Source: CAD feature listing. Evaluate the final solid. Frame: model axes, mm. Face numbers are marked on the shaded views. A direction names the side the tool comes from. Give positions to 0.01 mm unless a question says otherwise; leave off trailing zeros. Loops run counter-clockwise (first coordinate to the right, second up) from the corner with the lowest first, then second, coordinate; pieces in that order, holes last. Notation, with made-up numbers: M 22.25,66 L 46.25,66 A21 ccw 46.25,94 Z; hole C 89,88.25 d1. An arc over 180 degrees is marked long. Answer in a Markdown table with one row per item.
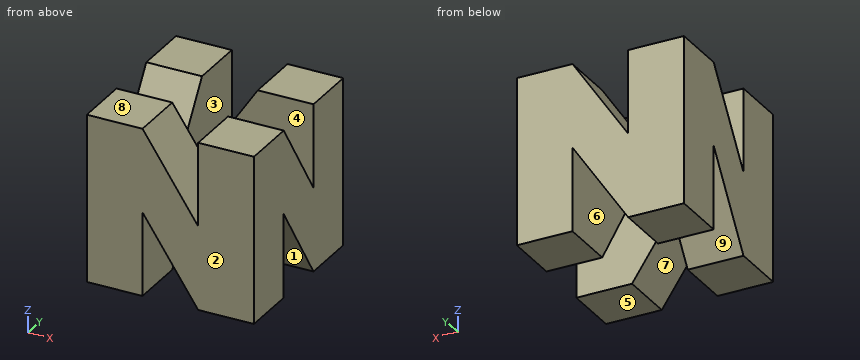
```python
from build123d import *

# Parameters (mm, degrees)
F0_W      = 152.4
F0_H      = 152.4
F1_DEPTH  = 76.2
F2_W      = 25.4
F2_H      = 25.4
F3_DEPTH  = 152.401
F5_DEPTH  = 50.8
F7_DEPTH  = 50.8
F9_DEPTH  = 50.8
F11_DEPTH = 50.8


with BuildPart() as f1:
    # F0 (on Top) → F1 (new body, symmetric)
    with BuildSketch(Plane.XY):
        with Locations((0, 4.4160668929)):
            Rectangle(F0_W, F0_H)
    extrude(amount=F1_DEPTH, both=True)

    # F2 (on face) → F3 (cut, through all)
    with BuildSketch(Plane.XY.offset(76.2)):
        Polygon((0, 29.8160668929), (-25.4, 29.8160668929), (0, 4.4160668929), align=None)
        with Locations((12.7, 17.1160668929)):
            Rectangle(F2_W, F2_H)
        Polygon((25.4, 4.4160668929), (0, 4.4160668929), (25.4, -20.9839331071), align=None)
        Polygon((25.4, -20.9839331071), (0, 4.4160668929), (0, -20.9839331071), align=None)
        with Locations((-12.7, -8.2839331071)):
            Rectangle(F2_W, F2_H)
        Polygon((0, 4.4160668929), (-25.4, 29.8160668929), (-25.4, 4.4160668929), align=None)
    extrude(amount=-F3_DEPTH, mode=Mode.SUBTRACT)

    # F4 (on face) → F5 (cut)
    with BuildSketch(Plane(origin=(0, 80.6160668929, 0), x_dir=(-1, 0, 0), z_dir=(0, 1, 0))):
        Polygon((25.4, -76.2), (-25.4, 0), (-25.4, -76.2), align=None)
        Polygon((25.4, 76.2), (-25.4, 76.2), (25.4, 0), align=None)
    extrude(amount=-F5_DEPTH, mode=Mode.SUBTRACT)

    # F6 (on face) → F7 (cut)
    with BuildSketch(Plane(origin=(-76.2, 0, 0), x_dir=(0, -1, 0), z_dir=(-1, 0, 0))):
        Polygon((20.9839331071, -76.2), (-29.8160668929, 0), (-29.8160668929, -76.2), align=None)
        Polygon((20.9839331071, 76.2), (-29.8160668929, 76.2), (20.9839331071, 0), align=None)
    extrude(amount=-F7_DEPTH, mode=Mode.SUBTRACT)

    # F8 (on face) → F9 (cut)
    with BuildSketch(Plane.XZ.offset(71.7839331071)):
        Polygon((25.4, -76.2), (-25.4, 0), (-25.4, -76.2), align=None)
        Polygon((25.4, 76.2), (-25.4, 76.2), (25.4, 0), align=None)
    extrude(amount=-F9_DEPTH, mode=Mode.SUBTRACT)

    # F10 (on face) → F11 (cut)
    with BuildSketch(Plane.YZ.offset(76.2)):
        Polygon((29.8160668929, -76.2), (-20.9839331071, 0), (-20.9839331071, -76.2), align=None)
        Polygon((29.8160668929, 76.2), (-20.9839331071, 76.2), (29.8160668929, 0), align=None)
    extrude(amount=-F11_DEPTH, mode=Mode.SUBTRACT)


solid = f1.part
```
Q1. Section query A-A (x = -2). Output: boundary loops of the cut face in (y, z).
Values follow:
| item | result |
|---|---|
| outline | M -71.78,-35.1 L -20.98,-35.1 L -20.98,41.1 L -71.78,41.1 Z; M 29.82,-41.1 L 80.62,-41.1 L 80.62,35.1 L 29.82,35.1 Z |
Q2. Section query D-D (x = 45.5). Output: boundary loops of the cut face in (y, z), plus the area to 3 significant figures.
Values follow:
| item | result |
|---|---|
| outline | M -71.78,-76.2 L -20.98,-76.2 L -20.98,0 L 29.82,-76.2 L 80.62,-76.2 L 80.62,76.2 L 29.82,76.2 L 29.82,0 L -20.98,76.2 L -71.78,76.2 Z |
| area | 19,400 mm^2 |
Q3. Contact query for flat-ended pins moving along their axis: pin 1 Ø3 at (x, y) = (-60.5, 20.5) entering from +Z; pin 2 Ø2 at (x, y) = (22.5, -35.5) entering from +Z. Output: stop coordinate, or through.
Values follow:
| item | result |
|---|---|
| pin 1 | z = 64.48 |
| pin 2 | z = 5.85 |
Q4. Reachability of the marked faces 5, 6, 7, 8 and 9 from +Z, -Z, +X, -X, +Y, -Y: full face, straight path, thin tool, end or side. Return the list, or none.
Values follow:
| item | result |
|---|---|
| face 5 | -Z, +X, -X, +Y, -Y |
| face 6 | none |
| face 7 | -Z, -Y |
| face 8 | +Z, +X, -X, +Y, -Y |
| face 9 | -Z, -X |
Q5. Mould query, pull axis Y, two halves, no side actions, for the marked faces 1, 2, 3 and 4. Classes: +Y half, -Y half, draft (parallel to the pull), parting line (faces both ways), or undercut.
Values follow:
| item | result |
|---|---|
| face 1 | undercut |
| face 2 | -Y half |
| face 3 | draft |
| face 4 | undercut |
Q6. Ray query, probe 1 along Y at (x, z) = (-13, -4.5); probe 2 along X at (y, z) = (7, -9); probe 3 along Y at (x, z) = (15, 51). Return the intervals inside material, ascending. Write a range as from..to.
Values follow:
| item | result |
|---|---|
| probe 1 | -71.78..-20.98, 29.82..80.62 |
| probe 2 | -76.2..-25.4, 25.4..76.2 |
| probe 3 | 29.82..80.62 |
Q7. Section query C-C (z = 8). Output: boundary loops of the cut face in (x, y).
Values follow:
| item | result |
|---|---|
| outline | M -76.2,-71.78 L 20.07,-71.78 L 20.07,-20.98 L -76.2,-20.98 Z; M -76.2,-15.65 L -25.4,-15.65 L -25.4,80.62 L -76.2,80.62 Z; M -20.07,29.82 L 76.2,29.82 L 76.2,80.62 L -20.07,80.62 Z; M 25.4,-71.78 L 76.2,-71.78 L 76.2,24.48 L 25.4,24.48 Z |
Q8. Section query B-B (y = -10.5). Output: boundary loops of the cut face in (x, z), plus the area to 3 significant figures.
Values follow:
| item | result |
|---|---|
| outline | M -76.2,-60.47 L -25.4,-60.47 L -25.4,15.73 L -76.2,15.73 Z; M 25.4,-15.73 L 76.2,-15.73 L 76.2,60.47 L 25.4,60.47 Z |
| area | 7,740 mm^2 |
